Geometry: see drawing. Coordinates: mm, zero at the bounding-box minimum. A direction names the side the tool comes from. Give positions to 0.01 mm unless a question says otherwise; leave off trailing zeros. Write each loop counter-clockwise with the first axis right and the second up, starting at its lowest first coordinate (ties: lowest second). Pieces come first, ordered by that corner, then holes. Notation, with made-up numbers: M 54.5,57 L 87.5,57 A8 ccw 87.5,64 Z; hole C -22.75,60.25 d4. An arc over 180 degrees is marked long. Use a Markdown table: item, result. Add a question column.
(1) Reachability of the marked faces 4 and 5 from +Z, -Z, +X, -X, +Y, -Y: full face, straight path, thin tool, end or side. Return the list, or none.
(2) Cut plane B-B (z = 8). Output: boundary loops of the cut face in (x, y).
(3) Cut plane C-C (x = 15). Output: boundary loops of the cut face in (y, z).
(4) Cut plane A-A (y = 17.5). Output: boundary loops of the cut face in (x, z), plus the area to 3 significant figures.
(5) Material intervals for L1, parallel to X at y = 7.75, z = 18.5; L2, parallel to Y at x = 14.25, z = 7.5; L3, parallel to Y at x = 9.25, z = 14.75, sorted ascending.
(6) Draft query along X for the marked faces 1, 2 and 3. Return one class per face: released by +X, released by -X, zero draft, split by the parting line, or undercut.
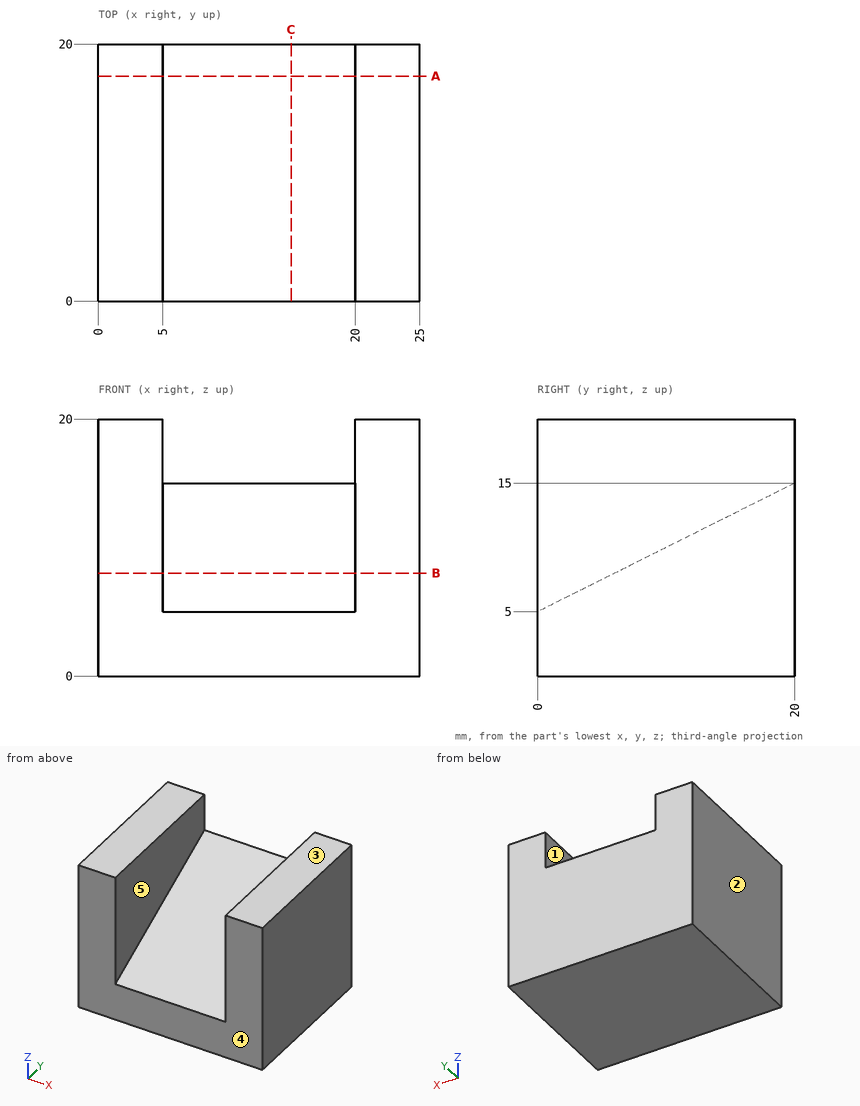
Answer list:
| question | item | result |
|---|---|---|
| 1 | face 4 | +Z, -Z, +X, -X, -Y |
| 1 | face 5 | +Z, -Y |
| 2 | outline | M 0,0 L 5,0 L 5,6 L 20,6 L 20,0 L 25,0 L 25,20 L 0,20 Z |
| 3 | outline | M 0,0 L 20,0 L 20,15 L 0,5 Z |
| 4 | outline | M 0,0 L 25,0 L 25,20 L 20,20 L 20,13.75 L 5,13.75 L 5,20 L 0,20 Z |
| 4 | area | 406 mm² |
| 5 | L1 | 0 to 5, 20 to 25 |
| 5 | L2 | 5 to 20 |
| 5 | L3 | 19.5 to 20 |
| 6 | face 1 | undercut |
| 6 | face 2 | released by -X |
| 6 | face 3 | zero draft |
